Build history of the part. All positions in model axes, mm. Face numbers are marked on the shaded views. A direction names the side the tool comes from. Round coordinates to 2 decimals unless told otherwise and drop trailing zeros. Write each loop counter-clockwise with the first axis right and the second up, starting at its lowest first coordinate (ties: lowest second). Pieces come first, ordered by that corner, then holes.
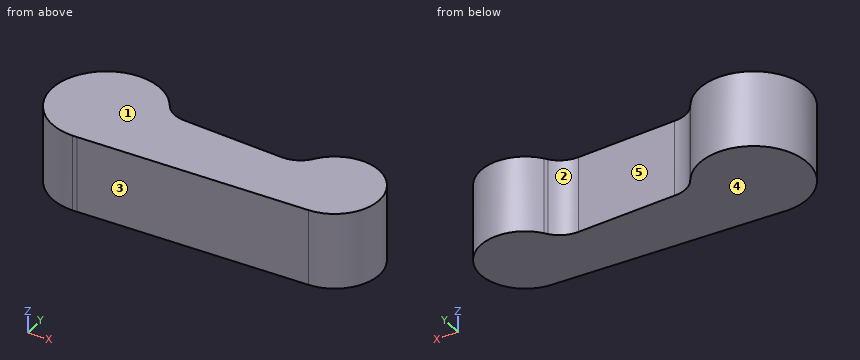
from build123d import *

# Parameters (mm, degrees)
F1_DEPTH = 132.5


with BuildPart() as f1:
    # F0 (on Top) → F1 (new body)
    with BuildSketch(Plane.XY):
        with BuildLine():
            ThreePointArc((75.866733, 55.4999), (78.237558, 51.506392), (80.968692, 47.750088))
            ThreePointArc((80.968692, 47.750088), (78.513391, 51.687982), (75.866733, 55.4999))
        make_face()
        with BuildLine():
            ThreePointArc((120, 29), (98.349314, 33.930633), (80.968692, 47.750088))
            ThreePointArc((80.968692, 47.750088), (78.237558, 51.506392), (75.866733, 55.4999))
            ThreePointArc((75.866733, 55.4999), (-83.824193, 42.538273), (0, -94))
            Line((0, -94), (7.711251, -93.683171))
            Line((7.711251, -93.683171), (403.181522, -77.434669))
            ThreePointArc((403.181522, -77.434669), (468.607926, 36.044451), (338.04126, 46.554963))
            ThreePointArc((338.04126, 46.554963), (336.236443, 43.723582), (334.245664, 41.019718))
            ThreePointArc((334.245664, 41.019718), (315.896852, 26.576201), (292.99007, 22.040415))
            Line((292.99007, 22.040415), (120, 29))
        make_face()
        with BuildLine():
            Line((7.711251, -93.683171), (0, -94))
            ThreePointArc((0, -94), (3.858878, -93.920759), (7.711251, -93.683171))
        make_face()
        with BuildLine():
            ThreePointArc((338.04126, 46.554963), (336.083514, 43.828448), (334.245664, 41.019718))
            ThreePointArc((334.245664, 41.019718), (336.236443, 43.723582), (338.04126, 46.554963))
        make_face()
    extrude(amount=-F1_DEPTH)


solid = f1.part
1) Wall check: L1, parallel to X at y = 3.5, z = -115; L2, parallel to X at y = 53, z = -36; L3, parallel to X at y = 38.5, z = -8. Give the ranges that are in metal, low to high.
Results:
L1: x = -93.93 to 477.42
L2: x = -77.63 to 77.63, 343.46 to 456.54
L3: x = -85.75 to 90.68, 332.12 to 467.26
2) Slice it at B-B (y = -52). Write the cut outline in (x, z).
Results:
outline: (-78.31, -132.5) - (457.47, -132.5) - (457.47, 0) - (-78.31, 0) - close
3) Mould opens along X. For the marked faces 3, 4 and 5 say: released by +X, released by -X, zero draft, split by the parting line, or undercut.
Results:
face 3: released by +X
face 4: zero draft
face 5: undercut
4) Which spindle directions (+Z, -Z, +X, -X, +Y, -Y) get a long thin tool onto all of the face, cutting with end or side? Do the marked faces 1 and 2. Say none if no direction does.
Results:
face 1: +Z, +X, -X, +Y, -Y
face 2: +Z, -Z, +Y
5) Slice it at A-A (z = -72). Write the cut outline in (x, y).
Results:
outline: (0, -94) arc R94 ccw to (7.71, -93.68) - (403.18, -77.43) arc R77.5 ccw (long way) to (338.04, 46.55) arc R77.5 ccw to (334.25, 41.02) arc R50 cw to (292.99, 22.04) - (120, 29) arc R50 cw to (80.97, 47.75) arc R94 ccw to (75.87, 55.5) arc R94 ccw (long way) to start
6) Slice it at C-C (x = 46.5). Write the cut outline in (y, z).
Results:
outline: (-92.09, -132.5) - (81.69, -132.5) - (81.69, 0) - (-92.09, 0) - close
7) Pin check, flat tips, straight feed: pin 1 Ø8 at (y, z) = (53, -60) entering from +X; pin 2 Ø3 at (x, z) = (140, -65) entering from +Y; pin 3 Ø2 at (x, z) = (160.5, -20) entering from +Y. Stop position of each tip, or through.
Results:
pin 1: stops at x = 460.04
pin 2: stops at y = 28.26
pin 3: stops at y = 27.41
